Geometry: final body of the model. Coordinates: model frame, mm. A direction names the side the tool comes from. Give positions to 0.01 mm unless a question says otherwise; leave off trailing zeros. Write each loop counter-clockwise with the first axis right and the second up, starting at its lowest first coordinate (ties: lowest second). Pieces come first, ordered by that corner, then holes. Notation, with made-up numbers: (71.25, -38) -> (76.25, -38) arc R28 cw to (76.25, -20) -> close; hole circle Ø5 at (83, -37). An arc over 180 degrees is marked (long way). Answer as a JSON object with one key per item and string values.
Autodesk Inventor part; units mm, degrees
ref_plane "YZ Plane" through (0, 0, 0) normal (1, 0, 0) x (0, 1, 0)
ref_plane "XZ Plane" through (0, 0, 0) normal (0, 1, 0) x (-1, 0, 0)
ref_plane "XY Plane" through (0, 0, 0) normal (0, 0, 1) x (1, 0, 0)
sketch "Sketch1" plane through (0, 0, 0) normal (0, 1, 0) x (-1, 0, 0)
  line L0 (0, 0) -> (56, 0)
  line L1 (56, 0) -> (56, -15)
  line L2 (56, -15) -> (0, -15)
  line L3 (0, -15) -> (0, 0)
  line L4 (59, 3) -> (-3, 3)
  line L5 (-3, 3) -> (-3, -18)
  line L6 (-3, -18) -> (59, -18)
  line L7 (59, -18) -> (59, 3)
  dimension "d0" = 56
  dimension "d1" = 15
  dimension "d2" = 3
  dimension "d3" = 3
  dimension "d4" = 3
  dimension "d5" = 3
extrude "Extrusion1" add sketch "Sketch1" along normal blind 2 contours L0 L1 L2 L3
extrude "Extrusion2" add sketch "Sketch1" along normal blind 17
sketch "Sketch2" plane through (0, 17, 0) normal (0, 1, 0) x (1, 0, 0)
  line L0 (-56, 15) -> (0, 15)
  line L1 (-59, 18) -> (-59, -3)
  line L2 (-56, 15) -> (-59, 15)
  line L3 (-59, 15) -> (-59, 0)
  line L4 (-59, 0) -> (-56, 0)
  line L5 (-56, 0) -> (-56, 15)
  point P0 (0, 0)
extrude "Extrusion3" cut sketch "Sketch2" against normal blind 2
fillet "Fillet1" radius 1.25 10 edges at (-29.5, 17, -15) (-29.5, 17, 0) (-28, 17, -18) (-28, 17, 3) (0, 17, -7.5) (3, 17, -7.5) (-59, 15, -7.5) (-56, 15, -7.5) (-59, 16, -15) (-59, 16, 0)
fillet "Fillet2" radius 1.25 12 edges at (-59, 16.6339, 2.6339) (-59, 17, 1.5) (-58.6339, 16.6339, 0.3661) (-59, 7.875, 3) (-59, 16.6339, -17.6339) (-59, 17, -16.5) (-58.6339, 16.6339, -15.3661) (-59, 7.875, -18) (2.6339, 16.6339, 2.6339) (3, 7.875, 3) (2.6339, 16.6339, -17.6339) (3, 7.875, -18)
properties part number "battery_compartment"
Q1. First-contact query: P1, Ø1, axis at x = -19.5, z = -10.5, coming from the +Y side. Flat tip, straight axial feed; report the tip coordinate or a pass-through.
Values:
{"P1": "y = 2"}
Q2. Material intervals for L1, parallel to Z at x = -33, y = 8.5; L2, parallel to X at y = 8.5, z = -8.5; L3, parallel to Y at x = -5, z = -6, sorted ascending. Write a range as from..to.
Values:
{"L1": "-18..-15, 0..3", "L2": "-59..-56, 0..3", "L3": "0..2"}
Q3. Set-up query: faces 4 (the flat face through (3, 8, -7)), 5 (the cylindrical face through (0.376, 16.644, -7.377)), 6 (the flat face through (-29, 9, 0)). Return all of +Z, -Z, +X, -X, +Y, -Y with unobstructed straight access to the full face (end or side cutting, diameter ignored); none if empty.
Values:
{"face 4": "+Z, -Z, +X, +Y, -Y", "face 5": "-X, +Y", "face 6": "+Y"}
Q4. Cut plane B-B (y = 9.75). Return the cut outline in (x, z).
Values:
{"outline": "(-59, -16.75) arc R1.25 ccw to (-57.75, -18) -> (1.75, -18) arc R1.25 ccw to (3, -16.75) -> (3, 1.75) arc R1.25 ccw to (1.75, 3) -> (-57.75, 3) arc R1.25 ccw to (-59, 1.75) -> close; hole (-56, -15) -> (0, -15) -> (0, 0) -> (-56, 0) -> close"}
Q5. Cut plane C-C (z = -7.25). Return the cut outline in (x, y).
Values:
{"outline": "(-59, 0) -> (3, 0) -> (3, 15.75) arc R1.25 ccw to (1.75, 17) -> (1.25, 17) arc R1.25 ccw to (0, 15.75) -> (0, 2) -> (-56, 2) -> (-56, 13.75) arc R1.25 ccw to (-57.25, 15) -> (-57.75, 15) arc R1.25 ccw to (-59, 13.75) -> close"}
Q6. Mould query, pull axis Z, two halves, no side actions, for faces 1 (the cylindrical face through (-56.376, 14.644, -7.605)), 2 (the flat face through (-28, 8, 3)), 3 (the cylindrical face through (2.624, 7.765, -17.644)). Classes: pulls with the +Z half, pulls with the -Z half, needs draft (parallel to the pull), parting line crosses it, or undercut.
Values:
{"face 1": "undercut", "face 2": "pulls with the +Z half", "face 3": "pulls with the -Z half"}
Q7. Cut plane A-A (x = -2.5). Return the cut outline in (y, z).
Values:
{"outline": "(0, -18) -> (15.75, -18) arc R1.25 ccw to (17, -16.75) -> (17, -16.25) arc R1.25 ccw to (15.75, -15) -> (2, -15) -> (2, 0) -> (15.75, 0) arc R1.25 ccw to (17, 1.25) -> (17, 1.75) arc R1.25 ccw to (15.75, 3) -> (0, 3) -> close"}
